Source: CAD feature listing. Evaluate the final solid. Frame: model axes, mm. Face numbers are marked on the shaded views. Round coordinates to 2 decimals unless told otherwise and drop trailing zeros. Loops run counter-clockwise (first coordinate to the right, second up) from the corner with the lowest first, then second, coordinate; pieces in that order, holes last.
(1) Mould query, pull axis X, two halves, no side actions, for the marked faces 1, 2 and 3. Classes: pulls with the +X half, pulls with the -X half, needs draft (parallel to the pull), parting line crosses it, or undercut.
(2) Section A-A, the plane x = -44. Return the cut outline in (y, z), plus the area to 3 significant figures.
(3) First-contact query: pin 1 Ø3 at (x, z) = (0.5, 2) entering from -Y; pin 2 Ø1 at (x, z) = (-15.5, 1) entering from -Y; pin 3 Ø2 at (y, z) = (-26, 3) entering from -X. Flat tips, straight axial feed; report the tip coordinate or a pass-through.
(4) Material intervals for probe 1 along Y at (x, z) = (-4.5, 1.75); probe 2 along X at (y, z) = (-17, 4.25); probe 3 along X at (y, z) = (8, 5.25), sorted ascending.
(5) Section C-C, the plane z = 3.25. Count the separate pieces of the cut face and the enclosed holes in it, plus the area to 3 significant figures.
(6) Section B-B, the plane y = 4. Return the cut outline in (x, z).
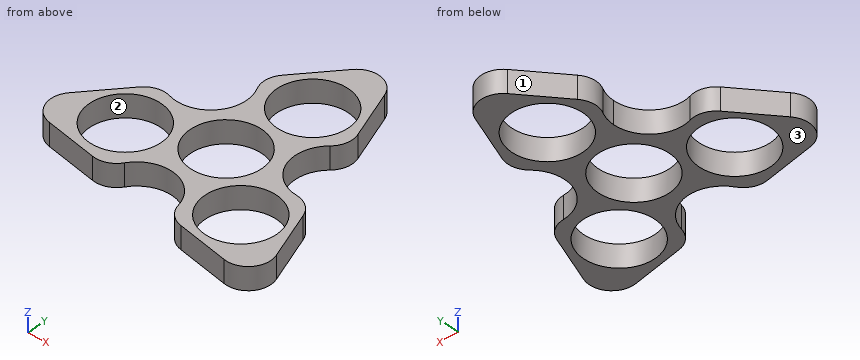
```python
from build123d import *

# Parameters (mm, degrees)
F0_R     = 11.1
F1_DEPTH = 7
F2_R     = 7


with BuildPart() as f1:
    # F0 (on Top) → F1 (new body)
    with BuildSketch(Plane.XY):
        with BuildLine():
            Line((-38.9624627261, -8.1840724655), (-60.7952496686, -34.2480210213))
            Line((-60.7952496686, -34.2480210213), (-27.306814625, -40.123794871))
            ThreePointArc((-27.306814625, -40.123794871), (-15.5182325204, -31.0662352189), (-5.4723209344, -42.0247805283))
            ThreePointArc((-5.4723209344, -42.0247805283), (-5.5137756251, -42.9788689424), (-5.6378272439, -43.9257661855))
            Line((-5.6378272439, -43.9257661855), (27.8506077997, -49.8015400352))
            Line((27.8506077997, -49.8015400352), (16.1949596986, -17.8618176297))
            ThreePointArc((16.1949596986, -17.8618176297), (2.090575123, -11.2993230017), (8.6530697509, 2.8050615739))
            Line((8.6530697509, 2.8050615739), (-3.0025783502, 34.7447839795))
            Line((-3.0025783502, 34.7447839795), (-24.8353652927, 8.6808354236))
            ThreePointArc((-24.8353652927, 8.6808354236), (-21.9314911759, 4.9013893297), (-20.8989140094, 0.2483814791))
            ThreePointArc((-20.8989140094, 0.2483814791), (-27.2459061587, -9.7190413544), (-38.9624627261, -8.1840724655))
        make_face()
        with Locations((-35.7535122499, -24.7765792781)):
            Circle(F0_R, mode=Mode.SUBTRACT)
        with Locations((7.3296251626, -32.6118866408)):
            Circle(F0_R, mode=Mode.SUBTRACT)
        with Locations((-11.9824067397, -16.4349256924)):
            Circle(F0_R, mode=Mode.SUBTRACT)
        with Locations((-7.6287635535, 8.378265008)):
            Circle(F0_R, mode=Mode.SUBTRACT)
    extrude(amount=F1_DEPTH)

    # F2
    f2_edges = [f1.edges().sort_by_distance(p)[0] for p in [
        (-3.002578, 34.744784, 3.5),
        (-24.835365, 8.680835, 3.5),
        (-38.962463, -8.184072, 3.5),
        (-60.79525, -34.248021, 3.5),
        (-27.306815, -40.123795, 3.5),
        (-5.637827, -43.925766, 3.5),
        (16.19496, -17.861818, 3.5),
        (8.65307, 2.805062, 3.5),
        (27.850608, -49.80154, 3.5),
    ]]
    fillet(f2_edges, radius=F2_R)


solid = f1.part
```
Output values:
1. face 1: pulls with the -X half
1. face 2: undercut
1. face 3: needs draft
2. outline: (-37.19, 0) - (-32.21, 0) - (-32.21, 7) - (-37.19, 7) - close; (-17.35, 0) - (-14.2, 0) - (-14.2, 7) - (-17.35, 7) - close
2. area: 57.0 mm2
3. pin 1: stops at y = -45.27
3. pin 2: stops at y = -31.12
3. pin 3: stops at x = -54.2
4. probe 1: y = -42.23 to -24.63, -8.24 to -2.27, 19.03 to 27.89
4. probe 2: x = -46.35 to -43.67, -27.83 to -23.07, -0.9 to 6.83
4. probe 3: x = -22.87 to -18.72, 3.46 to 6.76
5. separate pieces: 1
5. enclosed holes: 4
5. area: 1,260 mm2
6. outline: (-21.56, 0) - (-17.83, 0) - (-17.83, 7) - (-21.56, 7) - close; (2.57, 0) - (6.97, 0) - (6.97, 7) - (2.57, 7) - close
